Work out the finished part from the listing and answer in its coordinate system (mm). A direction names the side the tool comes from. Coordinates: 2 decimals unless noted, no trailing zeros. Order: outer loops, then holes, each group sorted by start corner. A loop starts at its lowest first (then second) coordinate and runs counter-clockwise, first axis right, second up. Notation, with made-up numbers: M -1,-12 L 21,-12 A19 ccw 21,2 Z; hole C -21,-5 d1. An arc over 180 degrees is marked long. Write item = value, one per line. Start each with the question number.
Q1. Find section C-C on z = 239.5. Give the vertices of the cut face in (x, y), and give its area (3 significant figures).
Q2. A tool of negligible diameter and unlimited length cuts with its end or side. For faces 1 (the flat face through (92, 306.185, 746)), 2 (the cylindrical face through (-49.3, 313.534, 246.288)), 3 (the flat face through (92, 164.604, 746)), 4 (the flat face through (187.178, 234, 746)), 5 (the flat face through (126.73, 457.98, 246.5)), from which of +Z, -Z, +X, -X, +Y, -Y can it reach the whole face along a straight path? Write none if from no direction.
Q3. Each of these flat-tipped pins is pushed along its axis until it touches: P1, Ø12, axis at x = 326.5, y = 254, coming from the +Z side; P2, Ø4, axis at x = 161, z = 317.5, coming from the -Y side; P3, Ø2, axis at y = 256.5, z = 84, coming from the -X side. Where does it stop, or does it pass through?
Q4. Find section B-B on x = 17. Give the vertices of the cut face in (y, z), and give its area (3 significant figures).
Q5. Find section A-A on y = 331.5. Give the vertices of the cut face in (x, z).
Q6. Straight lines are drawn through the part: line 1 along X through (y, z) = (233, 889); line 2 along Z through (x, y) = (132, 444); line 3 along Z through (x, y) = (87, 179). For each, find the intervals that lie inside material, in ascending order.
Q7. Find section D-D on y = 272.5. Give the vertices of the cut face in (x, z), and give its area (3 significant figures).
```python
from build123d import *

# Parameters (mm, degrees)
BOSS_EXTRU_1_DEPTH = 500
ESQUISSE2_W        = 187.1782881
ESQUISSE2_H        = 141.58126374
BOSS_EXTRU_2_DEPTH = 500
ESQUISSE3_R        = 76.59677213
BOSS_EXTRU_3_DEPTH = 100
BOSS_EXTRU_4_DEPTH = 50


with BuildPart() as part:
    # Esquisse1 → Boss.-Extru.1 (new body)
    with BuildSketch(Plane.XY):
        Polygon((0, 0), (0, 518.568521206), (257.06807621, 395.669035808), (174.541368625, -60.305866535), align=None)
    extrude(amount=BOSS_EXTRU_1_DEPTH)

    # Esquisse2 → Boss.-Extru.2 (add)
    with BuildSketch(Plane.XY.offset(500)):
        with Locations((93.58914405, 235.39430549)):
            Rectangle(ESQUISSE2_W, ESQUISSE2_H)
    extrude(amount=BOSS_EXTRU_2_DEPTH)

    # Esquisse3 → Boss.-Extru.3 (add)
    with BuildSketch(Plane.ZY):
        with Locations(Location((229.683047697, 238.758360313, 0), (0, 0, 180))):  # turned: the seam where the file's is
            Circle(ESQUISSE3_R)
    extrude(amount=BOSS_EXTRU_3_DEPTH)

    # Esquisse5 → Boss.-Extru.4 (add, symmetric)
    with BuildSketch(Plane(origin=(0, 306.18493736, 0), x_dir=(1, 0, 0), z_dir=(0, 1, 0))):
        Polygon((472.369351722, 254.21152486), (582.306234848, 125.789679085), (231.997079223, -174.096188988), (122.060196097, -45.674343213), align=None)
    extrude(amount=BOSS_EXTRU_4_DEPTH, both=True)


solid = part.part
```
Findings below:
q1.outline = M -100,162.79 L 0,162.79 L 0,0 L 174.54,-60.31 L 257.07,395.67 L 0,518.57 L 0,314.72 L -100,314.72 Z
q1.area = 124,000 mm^2
q2.face_1 = +Z, +X, -X, +Y
q2.face_2 = -X
q2.face_3 = +Z, +X, -X, -Y
q2.face_4 = +Z, +X, +Y, -Y
q2.face_5 = +Z, -Z, +X, +Y
q3.P1 = 97.98
q3.P2 = -56.32
q3.P3 = 0
q4.outline = M -5.87,0 L 510.44,0 L 510.44,500 L 306.18,500 L 306.18,1000 L 164.6,1000 L 164.6,500 L -5.87,500 Z
q4.area = 329,000 mm^2
q5.outline = M 0,0 L 175.41,0 L 472.37,-254.21 L 582.31,-125.79 L 245.45,162.58 L 245.45,500 L 0,500 Z
q6.line_1 = 0 to 187.18
q6.line_2 = 0 to 500
q6.line_3 = 0 to 1000
q7.outline = M -100,160.92 L 0,160.92 L 0,0 L 175.41,0 L 472.37,-254.21 L 582.31,-125.79 L 234.78,171.72 L 234.78,500 L 187.18,500 L 187.18,1000 L 0,1000 L 0,298.45 L -100,298.45 Z
q7.area = 291,000 mm^2
